Design review of the part built by this model. Coordinates are the model's own, in mm. A direction names the side the tool comes from. Give positions to 0.01 mm unless a question says otherwise; leave off trailing zeros. Loops run counter-clockwise (first coordinate to the right, second up) from the corner with the lowest first, then second, coordinate; pieces in that order, holes last. Notation, with made-up numbers: (-5.75, 11) -> (28.25, 11) arc R22 cw to (28.25, 49) -> close; hole circle Ø1 at (71, 53.5). An arc over 180 degrees is marked (long way). Answer in a Markdown table with one row per item. Add a question column.
(1) For line 1 (Y direction, x = -20, z = 25.95); line 2 (Y direction, x = -14, z = 24.5); line 3 (Y direction, x = -32.5, z = 1.5), list the stretches that pass through material, from the lowest coordinate up.
(2) Draft analysis for pull direction X (two halves, no side actions). For faces 1 (the flat face through (-48.221, -2.803, 24.437)), 2 (the flat face through (-3, -9.5, 25)), 3 (the flat face through (1, -27, 3)), 4 (the flat face through (-2, -17.5, 25)), state which applies: +X half, -X half, draft (parallel to the pull), parting line (faces both ways), or undercut.
(3) Consider section B-B on y = -13.5. Write out the cut boundary in (x, z), then the cut area to 3 significant figures.
(4) Consider section C-C on x = 29. Write out the cut boundary in (y, z).
(5) Consider section A-A on x = 0.5. Write out the cut boundary in (y, z), then the cut area to 3 significant figures.
(6) For pin 1 (1.8 mm diameter, centred on y = -28.5, z = 3, fed in from -X); pin 2 (1 mm diameter, centred on x = -27.5, y = -16, fed in from -Z); pin 3 (5 mm diameter, centred on y = 19, z = 17, fed in from -X), all flat-tipped, find the tip position at first contact; note any pin that passes through.
(7) Consider section D-D on z = 8.5. Write out the cut boundary in (x, y), then the cut area to 3 significant figures.
(8) For faces 5 (the cylindrical face through (19, 13.6, 25.5)), 6 (the flat face through (37, -2, 0)), 7 (the flat face through (1, -29, 6.3)), 8 (the flat face through (2, 27, 3)), list the 3-axis set-ups (+Z, -Z, +X, -X, +Y, -Y) from which the entire face can be reached by the end or side of a thin tool; tool diameter is ignored.
Autodesk Fusion 360 part; units mm, degrees
sketch "Sketch1" plane through (0, 0, 0) normal (0, 0, 1) x (1, 0, 0)
  line L0 (36, 27) -> (-36, 27)
  line L1 (-36, 27) -> (-36, -27)
  line L2 (-36, -27) -> (36, -27)
  line L3 (36, -27) -> (36, 27)
  line L4 (36, 30.6) -> (-36, 30.6)
  line L5 (-36, 35.6) -> (-36, -30.6)
  line L6 (-36, -30.6) -> (36, -30.6)
  line L7 (36, -30.6) -> (36, 30.6)
  line L8 (33, 35.6) -> (-36, 35.6)
  line L9 (41, -27.6) -> (41, 27.6)
  line L10 (33, -35.6) -> (-36, -35.6)
  line L11 (-36, -35.6) -> (-36, 30.6)
  arc A0 (41, 27.6) -> (33, 35.6) centre (33, 27.6) ccw
  arc A1 (33, -35.6) -> (41, -27.6) centre (33, -27.6) ccw
  circle A2 centre (-20, 0) radius 1.75
  circle A3 centre (15, 0) radius 1.75
  line L12 (-20, 9.5) -> (15, 9.5)
  arc A4 (15, 9.5) -> (15, 17.5) centre (15, 13.5) ccw
  line L13 (15, 17.5) -> (-20, 17.5)
  arc A5 (-20, 17.5) -> (-20, 9.5) centre (-20, 13.5) ccw
  line L14 (-20, 13.5) -> (15, 13.5) construction
  line L15 (1.75, 0) -> (22.5, 0)
  line L16 (-20, -9.5) -> (15, -9.5)
  line L17 (15, -17.5) -> (-20, -17.5)
  arc A6 (15, -17.5) -> (15, -9.5) centre (15, -13.5) ccw
  arc A7 (-20, -9.5) -> (-20, -17.5) centre (-20, -13.5) ccw
  dimension "d1" = 72
  dimension "d2" = 54
  dimension "d3" = 61.2
  dimension "d6" = 8
  dimension "d32" = 3.5
  dimension "d33" = 3.5
  dimension "d34" = 8
extrude "Extrude1" add sketch "Sketch1" along normal blind 6.3 contours L3 L4 L5 L6 L7 L8 L9 L10 L11 A0 A1 | L0 L4 L5 L7 L11 | L2 L5 L6 L7 L11
extrude "Extrude2" add sketch "Sketch1" along normal blind 24 contours L3 L4 L5 L6 L7 L8 L9 L10 L11 A0 A1
extrude "Extrude3" add sketch "Sketch1" along normal blind 27 and the other way blind -24
sketch "Sketch2" plane through (0, -35.6, 0) normal (0, -1, 0) x (1, 0, 0)
  line L0 (-36, 0) -> (33, 0)
  line L1 (33, 0) -> (33, 27)
  line L2 (-36, 27) -> (-36, 0)
  line L3 (-36, 0) -> (-49.5029, 27)
  line L4 (-36, 0) -> (-6, 0) construction
  line L5 (-36, 27) -> (-49.5029, 27)
  line L6 (33, 27) -> (-36, 27)
  line L7 (-36, 27) -> (-36, 24)
  line L8 (-36, 24) -> (-36.4845, 24)
  line L9 (-36.4845, 24) -> (-48.0026, 24)
  line L10 (-36, 0) -> (-36, 6.4)
  line L11 (-36, 6.4) -> (-36, 6)
  line L12 (-36, 6.4) -> (-39.2007, 6.4)
  line L13 (-36, 0) -> (-32.4, 0)
  line L14 (-49.5029, 27) -> (-47.5029, 27)
  line L15 (-36, 6.4) -> (-32.4, 6.4)
  line L16 (-32.4, 6.4) -> (-32.4, 0)
  dimension "d11" = 116.57
  dimension "d25" = 6.4
  dimension "d36" = 3.6
  dimension "d37" = 2
extrude "Extrude4" add sketch "Sketch2" against normal blind 5 contours L2 L3 L10 L11 L12 | L2 L3 L8 L9 L12
extrude "Extrude5" add sketch "Sketch2" along normal blind -71.2 and the other way blind 66.2 contours L2 L3 L10 L11 L12 | L2 L3 L8 L9 L12
extrude "Extrude6" add sketch "Sketch2" against normal blind 71.2 contours L2 L3 L5 L7 L8 L9 L14
extrude "Extrude7" cut sketch "Sketch2" along normal blind -8.6 and the other way blind 5 contours L0 L2 L10 L11 L13 L15 L16
extrude "Extrude8" cut sketch "Sketch2" along normal blind -66.2 and the other way blind 62.6 contours L0 L2 L10 L11 L13 L15 L16
chamfer "Chamfer1" distance 1 angle 45 2 edges at (-21.6316, 0.6328, 24) (13.3684, 0.6328, 24)
Values follow:
| question | item | result |
|---|---|---|
| 1 | line 1 | -35.6 to -17.5, -9.5 to -1.75, 1.75 to 9.5, 17.5 to 35.6 |
| 1 | line 2 | -35.6 to -17.5, -9.5 to 9.5, 17.5 to 35.6 |
| 1 | line 3 | -35.6 to -30.6, 30.6 to 35.6 |
| 2 | face 1 | -X half |
| 2 | face 2 | undercut |
| 2 | face 3 | draft |
| 2 | face 4 | undercut |
| 3 | outline | (-49.5, 27) -> (-48, 24) -> (-24, 24) -> (-24, 27) -> close; (19, 24) -> (36, 24) -> (36, 0) -> (41, 0) -> (41, 27) -> (19, 27) -> close |
| 3 | area | 260 mm2 |
| 4 | outline | (-35.6, 0) -> (-27, 0) -> (-27, 6.3) -> (-30.6, 6.3) -> (-30.6, 24) -> (30.6, 24) -> (30.6, 6.3) -> (27, 6.3) -> (27, 0) -> (35.6, 0) -> (35.6, 27) -> (-35.6, 27) -> close |
| 5 | outline | (-35.6, 0) -> (-27, 0) -> (-27, 6.3) -> (-30.6, 6.3) -> (-30.6, 24) -> (-17.5, 24) -> (-17.5, 27) -> (-35.6, 27) -> close; (-9.5, 24) -> (9.5, 24) -> (9.5, 27) -> (-9.5, 27) -> close; (17.5, 24) -> (30.6, 24) -> (30.6, 6.3) -> (27, 6.3) -> (27, 0) -> (35.6, 0) -> (35.6, 27) -> (17.5, 27) -> close |
| 5 | area | 451 mm2 |
| 6 | pin 1 | x = -32.4 |
| 6 | pin 2 | z = 24 |
| 6 | pin 3 | x = 36 |
| 7 | outline | (-40.25, -35.6) -> (33, -35.6) arc R8 ccw to (41, -27.6) -> (41, 27.6) arc R8 ccw to (33, 35.6) -> (-40.25, 35.6) -> (-40.25, 30.6) -> (36, 30.6) -> (36, -30.6) -> (-40.25, -30.6) -> close |
| 7 | area | 1,090 mm2 |
| 8 | face 5 | +Z, -Z |
| 8 | face 6 | -Z, +X, -X, +Y, -Y |
| 8 | face 7 | -X |
| 8 | face 8 | -Z, -X |
